Part model, mm, in its own coordinate system. A direction names the side the tool comes from. Give positions to 0.01 mm unless a question says otherwise; leave off trailing zeros. Order: outer loops, then holes, each group sorted by start corner. A loop starts at its lowest first (then second) coordinate and runs counter-clockwise, first axis right, second up.
1. Probe line 1 (Z direction, x = 27.5, y = 19) (3 decimals); line 2 (Z direction, x = 11, y = 45.5) (3 decimals); line 3 (X direction, y = 28.5, z = -59.5). List the from-to ranges inside material, lowest first.
2. Slice it at B-B on y = 30. List the corners of the cut face in (x, z) (3 decimals).
3. Slice it at D-D on x = 91. List the corners of the cut face in (y, z), and give its area (3 significant figures).
4. Mould opens along X. For faces 1 (the cylindrical face through (8.746, 7.009, -28.557)), 2 (the flat face through (39, 54, 55.88)), 3 (the flat face through (78.74, 54, 28)) say: +X half, -X half, draft (parallel to the pull), parting line (faces both ways), or undercut.
5. Drop flat-ended pins along their axis: pin 1 Ø3 at (x, z) = (23.5, 29) entering from -Y (3 decimals); pin 2 Ø14 at (y, z) = (54.5, 39.5) entering from +X; pin 3 Ø12 at (y, z) = (38.5, -72.5) entering from +X. Give the stop position or say it passes through.
6. Slice it at A-A on y = 19.5. List the corners of the cut face in (x, z) (3 decimals), and give its area (3 significant figures).
7. Which spindle directions (+Z, -Z, +X, -X, +Y, -Y) get a long thin tool onto all of the face, cutting with end or side? Do faces 4 (the flat face through (71, 30, -27.305)), 5 (the flat face through (38, 6, -4.064)), 6 (the flat face through (83, 60, -26.924)). Say none if no direction does.
8. Slice it at C-C on z = 43. List the corners of the cut face in (x, y) (3 decimals), and give its area (4 significant figures).
from build123d import *

# Parameters (mm, degrees)
SKETCH1_W           = 99.06
SKETCH1_H           = 27.305
SKETCH1_W_2         = 25.4
SKETCH1_H_2         = 4.445
BOSS_EXTRUDE1_DEPTH = 58.166
SKETCH2_R           = 3.175
CUT_EXTRUDE1_DEPTH  = 25.4
SKETCH3_R           = 30.7975
BOSS_EXTRUDE2_DEPTH = 101.6
SKETCH4_R           = 4.064
BOSS_EXTRUDE3_DEPTH = 2.54
BOSS_EXTRUDE4_DEPTH = 3.302
SKETCH6_W           = 58.42
SKETCH6_H           = 27.305
BOSS_EXTRUDE5_DEPTH = 2.159
SKETCH8_W           = 76.2
SKETCH8_H           = 4.064
CUT_EXTRUDE2_DEPTH  = 12.7
SKETCH9_W           = 78.74
SKETCH9_H           = 55.88
BOSS_EXTRUDE6_DEPTH = 12.7


with BuildPart() as part:
    # Sketch1 → Boss-Extrude1 (new body)
    with BuildSketch(Plane(origin=(0, 0, 0), x_dir=(1, 0, 0), z_dir=(0, 1, 0))):
        with Locations((49.53, 13.6525)):
            Rectangle(SKETCH1_W, SKETCH1_H)
        with Locations((86.36, 29.5275)):
            Rectangle(SKETCH1_W_2, SKETCH1_H_2)
    extrude(amount=BOSS_EXTRUDE1_DEPTH)

    # Sketch2 → Cut-Extrude1 (cut)
    with BuildSketch(Plane.XZ):
        with Locations(Location((39.878, -17.145, 0), (0, 0, 270))):
            Circle(SKETCH2_R)
    extrude(amount=-CUT_EXTRUDE1_DEPTH, mode=Mode.SUBTRACT)

    # Sketch3 → Boss-Extrude2 (add)
    with BuildSketch(Plane(origin=(0, 0, -27.305), x_dir=(-1, 0, 0), z_dir=(0, 0, -1))):
        with Locations(Location((-39.878, 29.845, 0), (0, 0, 113.134129644))):
            Circle(SKETCH3_R)
    extrude(amount=BOSS_EXTRUDE2_DEPTH)

    # Sketch4 → Boss-Extrude3 (add)
    with BuildSketch(Plane(origin=(0, 0, -27.305), x_dir=(-1, 0, 0), z_dir=(0, 0, -1))):
        with Locations((-11.938, 9.525)):
            Circle(SKETCH4_R)
    extrude(amount=BOSS_EXTRUDE3_DEPTH)

    # Sketch5 → Boss-Extrude4 (add)
    with BuildSketch(Plane(origin=(0, 58.166, 0), x_dir=(1, 0, 0), z_dir=(0, 1, 0))):
        with BuildLine():
            ThreePointArc((80.932762025, 22.479), (80.228633257, 24.915474366), (78.680076047, 26.924))
            ThreePointArc((78.680076047, 26.924), (76.342125496, 28.281267167), (73.66, 28.619482732))
            Line((73.66, 28.619482732), (73.66, 27.305))
            Line((73.66, 27.305), (70.125388313, 27.305))
            ThreePointArc((70.125388313, 27.305), (71.11041066, 15.776349905), (80.9625, 21.844))
            ThreePointArc((80.9625, 21.844), (80.955061434, 22.161847977), (80.932762025, 22.479))
        make_face()
        with BuildLine():
            Line((73.66, 27.305), (73.66, 28.619482732))
            ThreePointArc((73.66, 28.619482732), (71.799670865, 28.212378707), (70.125388313, 27.305))
            Line((70.125388313, 27.305), (73.66, 27.305))
        make_face()
        with BuildLine():
            Line((87.4395, 26.924), (78.680076047, 26.924))
            ThreePointArc((78.680076047, 26.924), (80.228633257, 24.915474366), (80.932762025, 22.479))
            Line((80.932762025, 22.479), (87.4395, 24.13))
            Line((87.4395, 24.13), (87.4395, 26.924))
        make_face()
    extrude(amount=BOSS_EXTRUDE4_DEPTH)

    # Sketch6 → Boss-Extrude5 (add)
    with BuildSketch(Plane(origin=(0, 58.166, 0), x_dir=(1, 0, 0), z_dir=(0, 1, 0))):
        with Locations((29.21, 13.6525)):
            Rectangle(SKETCH6_W, SKETCH6_H)
    extrude(amount=BOSS_EXTRUDE5_DEPTH)

    # Sketch8 → Cut-Extrude2 (cut)
    with BuildSketch(Plane.XZ):
        with Locations((38.1, -2.032)):
            Rectangle(SKETCH8_W, SKETCH8_H)
    extrude(amount=-CUT_EXTRUDE2_DEPTH, mode=Mode.SUBTRACT)

    # Sketch9 → Boss-Extrude6 (add)
    with BuildSketch(Plane(origin=(0, 60.325, 0), x_dir=(1, 0, 0), z_dir=(0, 1, 0))):
        with Locations((39.37, -27.94)):
            Rectangle(SKETCH9_W, SKETCH9_H)
    extrude(amount=-BOSS_EXTRUDE6_DEPTH)


solid = part.part
Data:
1. line 1: z = -128.905 to 0
1. line 2: z = -27.305 to 0
1. line 3: x = 9.11 to 70.65
2. outline: (0, -27.305) - (9.081, -27.305) - (9.081, -128.905) - (70.675, -128.905) - (70.675, -27.305) - (73.66, -27.305) - (73.66, -31.75) - (99.06, -31.75) - (99.06, 0) - (0, 0) - close
3. outline: (0, -31.75) - (58.17, -31.75) - (58.17, 0) - (0, 0) - close
3. area: 1,850 mm2
4. face 1: undercut
4. face 2: draft
4. face 3: +X half
5. pin 1: stops at y = 47.625
5. pin 2: stops at x = 78.74
5. pin 3: stops at x = 70.56
6. outline: (0, -27.305) - (10.87, -27.305) - (10.87, -128.905) - (68.886, -128.905) - (68.886, -27.305) - (73.66, -27.305) - (73.66, -31.75) - (99.06, -31.75) - (99.06, 0) - (0, 0) - close; hole circle Ø6.35 at (39.878, -17.145)
6. area: 8,680 mm2
7. face 4: -Z
7. face 5: +Z, -X, -Y
7. face 6: -Z, +X, +Y
8. outline: (0, 47.625) - (78.74, 47.625) - (78.74, 60.325) - (0, 60.325) - close
8. area: 1,000 mm2
